Here's how the part is built. I have some questions about the finished solid (model axes, mm). Face numbers are marked on the shaded views. A direction names the side the tool comes from. Coordinates: 2 decimals unless noted, no trailing zeros. Loops run counter-clockwise (first coordinate to the right, second up) from the corner with the lowest first, then second, coordinate; pieces in that order, holes last. Notation, with made-up numbers: (18.25, 64) -> (48.25, 64) arc R10 cw to (48.25, 72) -> close; hole circle Ø9 at (-17.5, 35.25). An arc over 180 degrees is marked (long way). Answer as a JSON object with one key per item and string values. Group by question number.
1) I want a section at B-B (y = -4.5). Write out the boundary of the cut face in (x, z), then the cut area to 3 significant figures.
2) I want a section at D-D (x = 13.75). Write out the boundary of the cut face in (y, z), then the cut area to 3 significant figures.
3) I want a section at A-A (y = 0). Write out the boundary of the cut face in (x, z) (3 decimals).
4) I want a section at C-C (z = 3.2). Count the separate pieces of the cut face and the enclosed holes in it, then the cut area to 3 significant figures.
5) If we mould it in two halves opening along X, with no side actions, what happens to the marked faces 1, 2 and 3? For each: +X half, -X half, draft (parallel to the pull), parting line (faces both ways), or undercut.
6) I'm going to push flat-ended pins straight in: pin 1 (3 mm diameter, centred on x = 8, z = 3.5, fed in from +Y); pin 2 (1.6 mm diameter, centred on y = -4, z = 3.5, fed in from +X); pin 3 (1 mm diameter, centred on y = 6.5, z = 2, fed in from +X); pin 4 (1.8 mm diameter, centred on y = -4.5, z = 3.2, fed in from -X). Where does each tip first touch, or does it pass through?
7) Which directions (+Z, -Z, +X, -X, +Y, -Y) give clear straight access to the entire face, cutting with the end or side of a thin tool? Please do the marked faces 4, 5, 6 and 7.
8) I need wall thicknesses on probe 1 along X at (y, z) = (-5.25, 2.5); probe 2 along Y at (x, z) = (-2.5, 3.25); probe 3 along Y at (x, z) = (10, 4.75). Which ranges of each line are inside material? Lowest first, please. Write a range as [from, to].
```python
from build123d import *

# Parameters (mm, degrees)
SKETCH_1_R           = 1.25
SKETCH_1_R_2         = 1.175
EXTRUDE_1_DEPTH      = 6.4
SKETCH_3_W           = 0.6
SKETCH_3_H           = 3.2
EXTRUDE_2_DEPTH      = 4
SKETCH_4_R           = 1
CUT_EXTRUDE_1_DEPTH  = 20
FILLET_1_R           = 1
FILLET_2_R           = 1
EXTRUDE_3_DEPTH      = 2
EXTRUDE_3_DEPTH_BACK = 2


with BuildPart() as part:
    # 草图1 → 凸台-拉伸1 (new body)
    with BuildSketch(Plane.XY):
        Polygon((-4.440828402, -2.5), (15.559171598, -2.5), (15.559171598, 7), (4.946745562, 7), (3.625739645, 7.7), (-4.440828402, 7.7), align=None)
        Circle(SKETCH_1_R, mode=Mode.SUBTRACT)
        with Locations((9.5, 0)):
            Circle(SKETCH_1_R_2, mode=Mode.SUBTRACT)
    extrude(amount=EXTRUDE_1_DEPTH)

    # 草图3 → 凸台-拉伸2 (add)
    with BuildSketch(Plane.XZ.offset(2.5)):
        with Locations((12.809171598, 3.2)):
            Rectangle(SKETCH_3_W, SKETCH_3_H)
        with Locations((-2.490828402, 3.2)):
            Rectangle(SKETCH_3_W, SKETCH_3_H)
        with Locations((5.509171598, 3.2)):
            Rectangle(SKETCH_3_W, SKETCH_3_H)
    extrude(amount=EXTRUDE_2_DEPTH)

    # 草图4 → 切除-拉伸1 (cut)
    with BuildSketch(Plane.ZY.offset(2.790828402)):
        with Locations((3.2, -4.5)):
            Circle(SKETCH_4_R)
    extrude(amount=-CUT_EXTRUDE_1_DEPTH, mode=Mode.SUBTRACT)

    # 圆角1
    fillet_1_edges = [part.edges().sort_by_distance(p)[0] for p in [
        (-2.490828402, -6.5, 1.6),
        (-2.490828402, -6.5, 4.8),
        (5.509171598, -6.5, 1.6),
        (5.509171598, -6.5, 4.8),
        (12.809171598, -6.5, 1.6),
        (12.809171598, -6.5, 4.8),
    ]]
    fillet(fillet_1_edges, radius=FILLET_1_R)

    # 圆角2
    fillet_2_edges = [part.edges().sort_by_distance(p)[0] for p in [
        (15.559171598, -2.5, 3.2),
        (-4.440828402, -2.5, 3.2),
        (15.559171598, 2.25, 6.4),
        (-4.440828402, 2.6, 6.4),
        (15.559171598, 2.25, 0),
        (5.559171598, -2.5, 0),
        (-4.440828402, 2.6, 0),
        (5.559171598, -2.5, 6.4),
    ]]
    fillet(fillet_2_edges, radius=FILLET_2_R)

    # 草图5 → 凸台-拉伸3 (add, two sides: drawn at the far end of the back side and taken through both)
    with BuildSketch(Plane.XY.offset(3.2).offset(-EXTRUDE_3_DEPTH_BACK)):
        with BuildLine():
            Line((0, 6.283577636), (0, 9.664597829))
            Line((0, 9.664597829), (17.8, 11.053189231))
            Line((17.8, 11.053189231), (17.8, 11.555466087))
            Line((17.8, 11.555466087), (17.585961229, 13.795738554))
            ThreePointArc((17.585961229, 13.795738554), (16.491955313, 14.447080857), (15.54107575, 13.60036733))
            Line((15.54107575, 13.60036733), (15.75254613, 11.386977345))
            Line((15.75254613, 11.386977345), (-0.5, 10.119103985))
            Line((-0.5, 10.119103985), (-0.5, 6.283577636))
            Line((-0.5, 6.283577636), (0, 6.283577636))
        make_face()
    extrude(amount=EXTRUDE_3_DEPTH + EXTRUDE_3_DEPTH_BACK)


solid = part.part
```
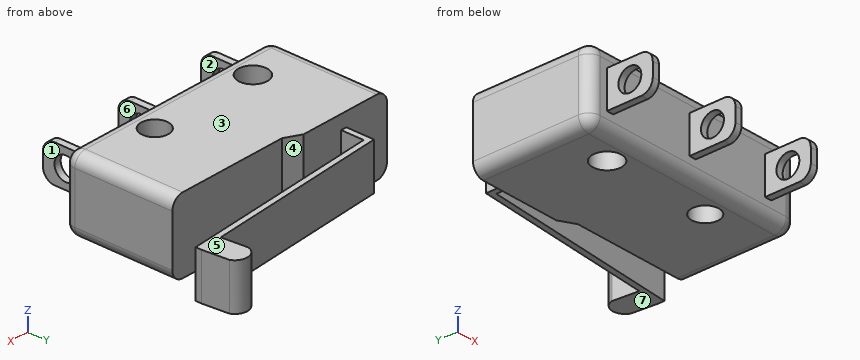
Determined:
{
 "1": {"outline": "(-2.79, 1.6) -> (-2.19, 1.6) -> (-2.19, 2.2) -> (-2.79, 2.2) -> close; (-2.79, 4.2) -> (-2.19, 4.2) -> (-2.19, 4.8) -> (-2.79, 4.8) -> close; (5.21, 1.6) -> (5.81, 1.6) -> (5.81, 2.2) -> (5.21, 2.2) -> close; (5.21, 4.2) -> (5.81, 4.2) -> (5.81, 4.8) -> (5.21, 4.8) -> close; (12.51, 1.6) -> (13.11, 1.6) -> (13.11, 2.2) -> (12.51, 2.2) -> close; (12.51, 4.2) -> (13.11, 4.2) -> (13.11, 4.8) -> (12.51, 4.8) -> close", "area": "2.16 mm^2"},
 "2": {"outline": "(-2.5, 1) arc R1 ccw to (-1.5, 0) -> (7, 0) -> (7, 6.4) -> (-1.5, 6.4) arc R1 ccw to (-2.5, 5.4) -> close; (10.74, 1.2) -> (11.23, 1.2) -> (11.23, 5.2) -> (10.74, 5.2) -> close", "area": "62.3 mm^2"},
 "3": {"outline": "(-4.441, 1) arc R1 ccw to (-3.441, 0) -> (-1.25, 0) -> (-1.25, 6.4) -> (-3.441, 6.4) arc R1 ccw to (-4.441, 5.4) -> close; (1.25, 0) -> (8.325, 0) -> (8.325, 6.4) -> (1.25, 6.4) -> close; (10.675, 0) -> (14.559, 0) arc R1 ccw to (15.559, 1) -> (15.559, 5.4) arc R1 ccw to (14.559, 6.4) -> (10.675, 6.4) -> close"},
 "4": {"separate pieces": "4", "enclosed holes": "2", "area": "206 mm^2"},
 "5": {"face 1": "+X half", "face 2": "undercut", "face 3": "draft"},
 "6": {"pin 1": "y = 10.9", "pin 2": "x = 13.11", "pin 3": "x = 15.56", "pin 4": "through"},
 "7": {"face 4": "+Z, -Z, +X", "face 5": "+Z, +X, -X, +Y", "face 6": "+Z, -Z, -Y", "face 7": "-Z, +X, -X, +Y"},
 "8": {"probe 1": "[-2.79, -2.19], [5.21, 5.81], [12.51, 13.11]", "probe 2": "[-6.5, -5.5], [-3.5, 7.7]", "probe 3": "[-2.5, -1.06], [1.06, 7], [10.44, 10.94]"}
}
